Work out the finished part from the listing and answer in its coordinate system (mm). Face numbers are marked on the shaded views. A direction names the side the tool comes from. Coordinates: 2 decimals unless noted, no trailing zeros. Order: outer loops, then holes, each group sorted by start corner. A loop starts at its lowest first (then second) coordinate and runs counter-clockwise, first axis right, second up. Notation, with made-up numbers: M 45.5,1 L 97.5,1 A24 ccw 97.5,22 Z; hole C -5.75,68.25 d5. An arc over 180 degrees is marked long. Use a Markdown table: item, result.
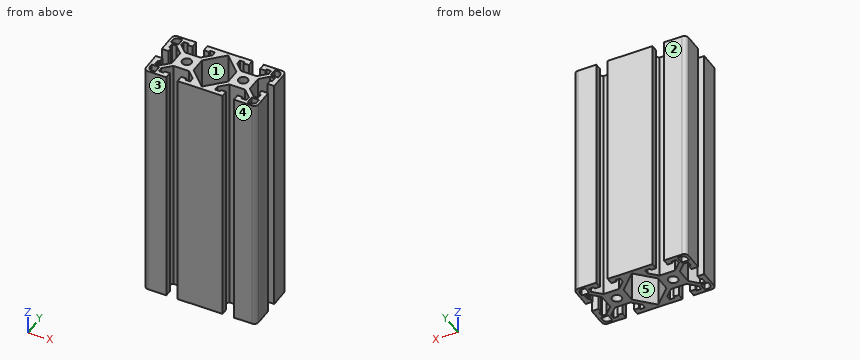
from build123d import *

# Parameters (mm, degrees)
SKETCH2_R                            = 3.35
F_40_SERIES_TS40_80LM_650037_1_DEPTH = 175
M8X1_25_TAPPED_HOLE1_D               = 6.8
M8X1_25_TAPPED_HOLE1_DEPTH           = 30
M8X1_25_TAPPED_HOLE1_TIP             = 2.042926105


with BuildPart() as part:
    # Sketch2 → 40 series TS40-80LM-650037(1) (new body)
    with BuildSketch(Plane(origin=(0, 0, 0), x_dir=(0, 1, 0), z_dir=(0, 0, 1))):
        with BuildLine():
            Line((0, -27.681), (-5.525738531, -27.681))
            Line((-5.525738531, -27.681), (-11.176, -33.331261469))
            Line((-11.176, -33.331261469), (-11.176, -36.6218))
            Line((-11.176, -36.6218), (-7.6835, -36.6218))
            Line((-7.6835, -36.6218), (-7.6835, -35.2248))
            Line((-7.6835, -35.2248), (-4.0488, -35.2248))
            Line((-4.0488, -35.2248), (-4.0488, -40))
            Line((-4.0488, -40), (-17, -40))
            ThreePointArc((-17, -40), (-19.121320344, -39.121320344), (-20, -37))
            Line((-20, -37), (-20, -24.0488))
            Line((-20, -24.0488), (-15.2248, -24.0488))
            Line((-15.2248, -24.0488), (-15.2248, -27.6835))
            Line((-15.2248, -27.6835), (-16.6218, -27.6835))
            Line((-16.6218, -27.6835), (-16.6218, -31.176))
            Line((-16.6218, -31.176), (-13.331261469, -31.176))
            Line((-13.331261469, -31.176), (-7.681, -25.525738531))
            Line((-7.681, -25.525738531), (-7.681, -20))
            Line((-7.681, -20), (-7.681, -14.474261469))
            Line((-7.681, -14.474261469), (-13.331261469, -8.824))
            Line((-13.331261469, -8.824), (-16.6218, -8.824))
            Line((-16.6218, -8.824), (-16.6218, -12.3165))
            Line((-16.6218, -12.3165), (-15.2248, -12.3165))
            Line((-15.2248, -12.3165), (-15.2248, -15.9512))
            Line((-15.2248, -15.9512), (-20, -15.9512))
            Line((-20, -15.9512), (-20, 15.9512))
            Line((-20, 15.9512), (-15.2248, 15.9512))
            Line((-15.2248, 15.9512), (-15.2248, 12.3165))
            Line((-15.2248, 12.3165), (-16.6218, 12.3165))
            Line((-16.6218, 12.3165), (-16.6218, 8.824))
            Line((-16.6218, 8.824), (-13.331261469, 8.824))
            Line((-13.331261469, 8.824), (-7.681, 14.474261469))
            Line((-7.681, 14.474261469), (-7.681, 25.525738531))
            Line((-7.681, 25.525738531), (-13.331261469, 31.176))
            Line((-13.331261469, 31.176), (-16.6218, 31.176))
            Line((-16.6218, 31.176), (-16.6218, 27.6835))
            Line((-16.6218, 27.6835), (-15.2248, 27.6835))
            Line((-15.2248, 27.6835), (-15.2248, 24.0488))
            Line((-15.2248, 24.0488), (-20, 24.0488))
            Line((-20, 24.0488), (-20, 37))
            ThreePointArc((-20, 37), (-19.121320344, 39.121320344), (-17, 40))
            Line((-17, 40), (-4.0488, 40))
            Line((-4.0488, 40), (-4.0488, 35.2248))
            Line((-4.0488, 35.2248), (-7.6835, 35.2248))
            Line((-7.6835, 35.2248), (-7.6835, 36.6218))
            Line((-7.6835, 36.6218), (-11.176, 36.6218))
            Line((-11.176, 36.6218), (-11.176, 33.331261469))
            Line((-11.176, 33.331261469), (-5.525738531, 27.681))
            Line((-5.525738531, 27.681), (0, 27.681))
            Line((0, 27.681), (5.525738531, 27.681))
            Line((5.525738531, 27.681), (11.176, 33.331261469))
            Line((11.176, 33.331261469), (11.176, 36.6218))
            Line((11.176, 36.6218), (7.6835, 36.6218))
            Line((7.6835, 36.6218), (7.6835, 35.2248))
            Line((7.6835, 35.2248), (4.0488, 35.2248))
            Line((4.0488, 35.2248), (4.0488, 40))
            Line((4.0488, 40), (17, 40))
            ThreePointArc((17, 40), (19.121320344, 39.121320344), (20, 37))
            Line((20, 37), (20, 24.0488))
            Line((20, 24.0488), (15.2248, 24.0488))
            Line((15.2248, 24.0488), (15.2248, 27.6835))
            Line((15.2248, 27.6835), (16.6218, 27.6835))
            Line((16.6218, 27.6835), (16.6218, 31.176))
            Line((16.6218, 31.176), (13.331261469, 31.176))
            Line((13.331261469, 31.176), (7.681, 25.525738531))
            Line((7.681, 25.525738531), (7.681, 20))
            Line((7.681, 20), (7.681, 14.474261469))
            Line((7.681, 14.474261469), (13.331261469, 8.824))
            Line((13.331261469, 8.824), (16.6218, 8.824))
            Line((16.6218, 8.824), (16.6218, 12.3165))
            Line((16.6218, 12.3165), (15.2248, 12.3165))
            Line((15.2248, 12.3165), (15.2248, 15.9512))
            Line((15.2248, 15.9512), (20, 15.9512))
            Line((20, 15.9512), (20, -15.9512))
            Line((20, -15.9512), (15.2248, -15.9512))
            Line((15.2248, -15.9512), (15.2248, -12.3165))
            Line((15.2248, -12.3165), (16.6218, -12.3165))
            Line((16.6218, -12.3165), (16.6218, -8.824))
            Line((16.6218, -8.824), (13.331261469, -8.824))
            Line((13.331261469, -8.824), (7.681, -14.474261469))
            Line((7.681, -14.474261469), (7.681, -20))
            Line((7.681, -20), (7.681, -25.525738531))
            Line((7.681, -25.525738531), (13.331261469, -31.176))
            Line((13.331261469, -31.176), (16.6218, -31.176))
            Line((16.6218, -31.176), (16.6218, -27.6835))
            Line((16.6218, -27.6835), (15.2248, -27.6835))
            Line((15.2248, -27.6835), (15.2248, -24.0488))
            Line((15.2248, -24.0488), (20, -24.0488))
            Line((20, -24.0488), (20, -37))
            ThreePointArc((20, -37), (19.121320344, -39.121320344), (17, -40))
            Line((17, -40), (4.0488, -40))
            Line((4.0488, -40), (4.0488, -35.2248))
            Line((4.0488, -35.2248), (7.6835, -35.2248))
            Line((7.6835, -35.2248), (7.6835, -36.6218))
            Line((7.6835, -36.6218), (11.176, -36.6218))
            Line((11.176, -36.6218), (11.176, -33.331261469))
            Line((11.176, -33.331261469), (5.525738531, -27.681))
            Line((5.525738531, -27.681), (0, -27.681))
        make_face()
        with Locations((0, -20)):
            Circle(SKETCH2_R, mode=Mode.SUBTRACT)
        with Locations((0, 20)):
            Circle(SKETCH2_R, mode=Mode.SUBTRACT)
        Polygon((-5.525738531, 12.319), (-17.844738531, 0), (-5.525738531, -12.319), (0, -12.319), (5.525738531, -12.319), (17.844738531, 0), (5.525738531, 12.319), (0, 12.319), align=None, mode=Mode.SUBTRACT)
        with BuildLine():
            Line((12.8372, 38.222), (12.8372, 32.8372))
            Line((12.8372, 32.8372), (18.222, 32.8372))
            Line((18.222, 32.8372), (18.222, 35.428))
            ThreePointArc((18.222, 35.428), (17.403656347, 37.403656347), (15.428, 38.222))
            Line((15.428, 38.222), (12.8372, 38.222))
        make_face(mode=Mode.SUBTRACT)
        with BuildLine():
            Line((12.8372, -32.8372), (18.222, -32.8372))
            Line((18.222, -32.8372), (18.222, -35.428))
            ThreePointArc((18.222, -35.428), (17.403656347, -37.403656347), (15.428, -38.222))
            Line((15.428, -38.222), (12.8372, -38.222))
            Line((12.8372, -38.222), (12.8372, -32.8372))
        make_face(mode=Mode.SUBTRACT)
        with BuildLine():
            Line((-12.8372, -38.222), (-12.8372, -32.8372))
            Line((-12.8372, -32.8372), (-18.222, -32.8372))
            Line((-18.222, -32.8372), (-18.222, -35.428))
            ThreePointArc((-18.222, -35.428), (-17.403656347, -37.403656347), (-15.428, -38.222))
            Line((-15.428, -38.222), (-12.8372, -38.222))
        make_face(mode=Mode.SUBTRACT)
        with BuildLine():
            Line((-18.222, 35.428), (-18.222, 32.8372))
            Line((-18.222, 32.8372), (-12.8372, 32.8372))
            Line((-12.8372, 32.8372), (-12.8372, 38.222))
            Line((-12.8372, 38.222), (-15.428, 38.222))
            ThreePointArc((-15.428, 38.222), (-17.403656347, 37.403656347), (-18.222, 35.428))
        make_face(mode=Mode.SUBTRACT)
    extrude(amount=F_40_SERIES_TS40_80LM_650037_1_DEPTH)

    # M8x1.25 Tapped Hole1
    with Locations(Plane(origin=(0, 0, 0), x_dir=(-1, 0, 0), z_dir=(0, 0, -1))):
        with Locations((-20, 0), (20, 0)):
            Hole(M8X1_25_TAPPED_HOLE1_D / 2, depth=M8X1_25_TAPPED_HOLE1_DEPTH)
            with Locations((0, 0, -(M8X1_25_TAPPED_HOLE1_DEPTH + M8X1_25_TAPPED_HOLE1_TIP / 2))):  # 118° drill point
                Cone(0, M8X1_25_TAPPED_HOLE1_D / 2, M8X1_25_TAPPED_HOLE1_TIP, mode=Mode.SUBTRACT)


solid = part.part
(1) A cutting plane is placed at A-A (y = 0). Determine the outline of the cut face in (x, z), then the cut area to 3 significant figures.
Conclusion:
| item | result |
|---|---|
| outline | M -27.68,0 L -23.4,0 L -23.4,30 L -23.35,30.03 L -23.35,175 L -27.68,175 Z; M -16.65,30.03 L -16.6,30 L -16.6,0 L -12.32,0 L -12.32,175 L -16.65,175 Z; M 12.32,0 L 16.6,0 L 16.6,30 L 16.65,30.03 L 16.65,175 L 12.32,175 Z; M 23.35,30.03 L 23.4,30 L 23.4,0 L 27.68,0 L 27.68,175 L 23.35,175 Z |
| area | 3,030 mm2 |
(2) A cutting plane is placed at C-C (z = 135.5). Give the number of separate pieces and of enclosed holes in the cut face, then the cut area to 3 significant figures.
Conclusion:
| item | result |
|---|---|
| separate pieces | 1 |
| enclosed holes | 7 |
| area | 1,330 mm2 |
(3) Given P1, Ø3.5, axis at x = -21.5, z = 46, coming from the -Y side; P2, Ø3, axis at y = 0, z = 106, coming from the -X side; P3, Ø2.5, axis at x = 38.5, z = 82, coming from the -Y side, each flat-ended and moving along its own axis, determine where each tip first touches the part or whether it passes through.
Conclusion:
| item | result |
|---|---|
| P1 | y = -7.68 |
| P2 | x = -27.68 |
| P3 | y = -19.99 |
(4) A cutting plane is placed at B-B (x = 20). Determine the outline of the cut face in (y, z), then the cut area to 3 significant figures.
Conclusion:
| item | result |
|---|---|
| outline | M -7.68,0 L -3.4,0 L -3.4,30 L -3.35,30.03 L -3.35,175 L -7.68,175 Z; M 3.35,30.03 L 3.4,30 L 3.4,0 L 7.68,0 L 7.68,175 L 3.35,175 Z |
| area | 1,510 mm2 |
(5) A cutting plane is placed at D-D (x = -2.5). Determine the outline of the cut face in (y, z).
Conclusion:
| item | result |
|---|---|
| outline | M -20,0 L -15.34,0 L -15.34,175 L -20,175 Z; M 15.34,0 L 20,0 L 20,175 L 15.34,175 Z |
(6) Which of the six approach directions +Z, -Z, +X, -X, +Y, -Y give full straight-line access (tool end or side, diameter ignored) to the marked faces 4 and 5?
Conclusion:
| item | result |
|---|---|
| face 4 | +Z, -Z, +X, -X, -Y |
| face 5 | +Z, -Z |
(7) Determine the mould class of the marked faces 1, 2 and 3 for opening direction Y: pulls with the +Y half, pulls with the -Y half, needs draft (parallel to the pull), parting line crosses it, or undercut.
Conclusion:
| item | result |
|---|---|
| face 1 | undercut |
| face 2 | pulls with the +Y half |
| face 3 | pulls with the -Y half |
(8) Straight lines are drawn through the part: L1, parallel to X at y = 0, z = 66.5; L2, parallel to Y at x = 15, z = 125.5; L3, parallel to X at y = 0, z = 23. For each, find the intervals that lie inside material, in ascending order.
Conclusion:
| item | result |
|---|---|
| L1 | -27.68 to -23.35, -16.65 to -12.32, 12.32 to 16.65, 23.35 to 27.68 |
| L2 | -20 to -15.22, -7.68 to 7.68, 15.22 to 20 |
| L3 | -27.68 to -23.4, -16.6 to -12.32, 12.32 to 16.6, 23.4 to 27.68 |
